Geometry check sheet. Reference: the model listing, model coordinates, mm. Face numbers are marked on the shaded views. A direction names the side the tool comes from. Coordinates: 2 decimals unless noted, no trailing zeros. Loops run counter-clockwise (first coordinate to the right, second up) from the corner with the lowest first, then second, coordinate; pieces in that order, holes last.
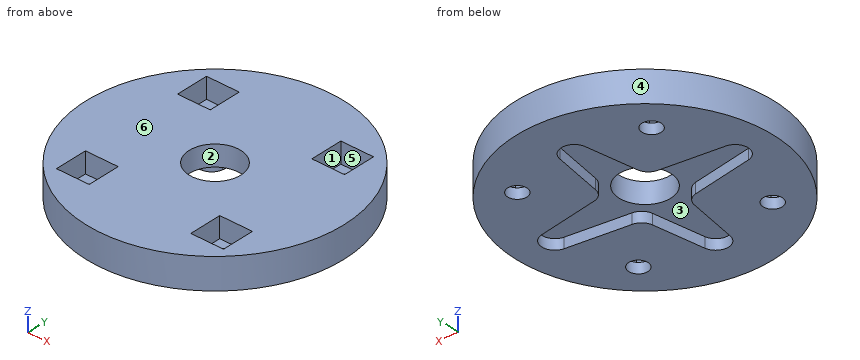
from build123d import *

# Parameters (mm, degrees)
BOSS_EXTRUDE1_OUTLINE_R = 25
BOSS_EXTRUDE1_DEPTH     = 2
SKETCH4_R               = 25
SKETCH4_R_2             = 5
BOSS_EXTRUDE2_DEPTH     = 4
SKETCH5_R               = 1.85
CUT_EXTRUDE1_DEPTH      = 36.860842154
SKETCH6_R               = 3
CUT_EXTRUDE2_DEPTH      = 4
SKETCH7_W               = 6.35
SKETCH7_H               = 6.35
CUT_EXTRUDE3_DEPTH      = 4


# Read off the part's stored shape, not the designer's step: Boss-Extrude1
with BuildPart() as part:
    # Boss-Extrude1 outline → Boss-Extrude1 (new body)
    with BuildSketch(Plane.XY):
        Circle(BOSS_EXTRUDE1_OUTLINE_R)
        with BuildLine():
            ThreePointArc((4.047481829, 6.234173406), (4.763543773, 4.853224592), (6.157606479, 4.163040916))
            Line((6.157606479, 4.163040916), (17.857142857, 2.474358297))
            ThreePointArc((17.857142857, 2.474358297), (20, 0), (17.857142857, -2.474358297))
            Line((17.857142857, -2.474358297), (6.157606479, -4.163040916))
            ThreePointArc((6.157606479, -4.163040916), (4.763543773, -4.853224592), (4.047481829, -6.234173406))
            Line((4.047481829, -6.234173406), (2.467267507, -15.903225806))
            ThreePointArc((2.467267507, -15.903225806), (0, -18), (-2.467267507, -15.903225806))
            Line((-2.467267507, -15.903225806), (-4.047481829, -6.234173406))
            ThreePointArc((-4.047481829, -6.234173406), (-4.763543773, -4.853224592), (-6.157606479, -4.163040916))
            Line((-6.157606479, -4.163040916), (-17.857142857, -2.474358297))
            ThreePointArc((-17.857142857, -2.474358297), (-20, 0), (-17.857142857, 2.474358297))
            Line((-17.857142857, 2.474358297), (-6.157606479, 4.163040916))
            ThreePointArc((-6.157606479, 4.163040916), (-4.763543773, 4.853224592), (-4.047481829, 6.234173406))
            Line((-4.047481829, 6.234173406), (-2.467267507, 15.903225806))
            ThreePointArc((-2.467267507, 15.903225806), (0, 18), (2.467267507, 15.903225806))
            Line((2.467267507, 15.903225806), (4.047481829, 6.234173406))
        make_face(mode=Mode.SUBTRACT)
    extrude(amount=BOSS_EXTRUDE1_DEPTH)

    # Sketch4 → Boss-Extrude2 (add)
    with BuildSketch(Plane.XY.offset(2)):
        Circle(SKETCH4_R)
        Circle(SKETCH4_R_2, mode=Mode.SUBTRACT)
    extrude(amount=BOSS_EXTRUDE2_DEPTH)

    # Sketch5 → Cut-Extrude1 (cut, through all)
    with BuildSketch(Plane.XY.offset(6)):
        with Locations((13.029498672, 13.274798425)):
            Circle(SKETCH5_R)
        with Locations((-13.029498672, 13.274798425)):
            Circle(SKETCH5_R)
        with Locations((-13.029498672, -13.274798425)):
            Circle(SKETCH5_R)
        with Locations((13.029498672, -13.274798425)):
            Circle(SKETCH5_R)
    extrude(amount=-CUT_EXTRUDE1_DEPTH, mode=Mode.SUBTRACT)

    # Sketch6 → Cut-Extrude2 (cut)
    with BuildSketch(Plane.XY.offset(6)):
        with Locations((-13.029498672, -13.274798425)):
            Circle(SKETCH6_R)
        with Locations((13.029498672, -13.274798425)):
            Circle(SKETCH6_R)
        with Locations((13.029498672, 13.274798425)):
            Circle(SKETCH6_R)
        with Locations((-13.029498672, 13.274798425)):
            Circle(SKETCH6_R)
    extrude(amount=-CUT_EXTRUDE2_DEPTH, mode=Mode.SUBTRACT)

    # Sketch7 → Cut-Extrude3 (cut)
    with BuildSketch(Plane.XY.offset(6)):
        with Locations((13.029498672, 13.274798425)):
            Rectangle(SKETCH7_W, SKETCH7_H)
        with Locations((13.029498672, -13.274798425)):
            Rectangle(SKETCH7_W, SKETCH7_H)
        with Locations((-13.029498672, -13.274798425)):
            Rectangle(SKETCH7_W, SKETCH7_H)
        with Locations((-13.029498672, 13.274798425)):
            Rectangle(SKETCH7_W, SKETCH7_H)
    extrude(amount=-CUT_EXTRUDE3_DEPTH, mode=Mode.SUBTRACT)


solid = part.part
1) Mould release check, pull along Y, two halves, no side actions. Record for the marked faces 4, 5 and 6: +Y half, -Y half, draft (parallel to the pull), parting line (faces both ways), or undercut.
Data:
face 4: parting line
face 5: undercut
face 6: draft
2) Section check D-D on y = -8.5. Record the cut outline in (x, z), and give its area (3 significant figures).
Data:
outline: (-23.51, 0) - (-3.68, 0) - (-3.68, 2) - (3.68, 2) - (3.68, 0) - (23.51, 0) - (23.51, 6) - (-23.51, 6) - close
area: 267 mm2
3) Section check C-C on z = 4.3. Record the cut outline in (x, y), and give its area (3 significant figures).
Data:
outline: circle Ø50 at (0, 0); hole (-16.2, -16.45) - (-9.85, -16.45) - (-9.85, -10.1) - (-16.2, -10.1) - close; hole (-16.2, 10.1) - (-9.85, 10.1) - (-9.85, 16.45) - (-16.2, 16.45) - close; hole circle Ø10 at (0, 0); hole (9.85, -16.45) - (16.2, -16.45) - (16.2, -10.1) - (9.85, -10.1) - close; hole (9.85, 10.1) - (16.2, 10.1) - (16.2, 16.45) - (9.85, 16.45) - close
area: 1,720 mm2
4) Depth check by flat-ended pin: pin 1 (2 mm diameter, centred on x = -17, y = 17, fed in from -Z); pin 2 (3 mm diameter, centred on y = -12, z = 3.5, fed in from +X); pin 3 (3 mm diameter, centred on x = -13.03, y = -13.27, fed in from +Z); pin 4 (5 mm diameter, centred on x = -13, y = 13, fed in from +Z). Enter the tip coordinate at first touch or a pass-through.
Data:
pin 1: stops at z = 0
pin 2: stops at x = 22.69
pin 3: passes through
pin 4: stops at z = 2
5) Section check A-A on y = 0. Record the cut outline in (x, z).
Data:
outline: (-25, 0) - (-20, 0) - (-20, 2) - (-5, 2) - (-5, 6) - (-25, 6) - close; (5, 2) - (20, 2) - (20, 0) - (25, 0) - (25, 6) - (5, 6) - close
6) Access from +Z, -Z, +X, -X, +Y, -Y to the whole of each face (thin tool, end or side, straight path). Record for the marked faces 1, 2 and 3.
Data:
face 1: +Z
face 2: +Z, -Z
face 3: -Z
7) Section check B-B on x = 0. Record the cut outline in (y, z).
Data:
outline: (-25, 0) - (-18, 0) - (-18, 2) - (-5, 2) - (-5, 6) - (-25, 6) - close; (5, 2) - (18, 2) - (18, 0) - (25, 0) - (25, 6) - (5, 6) - close
8) Material ranges on probe 1 along Y at (x, z) = (-13, 3.35); probe 2 along Y at (x, z) = (12, 1.1); probe 3 along Z at (x, y) = (-16, 2), recorded low to high.
Data:
probe 1: y = -21.35 to -16.45, -10.1 to 10.1, 16.45 to 21.35
probe 2: y = -21.93 to -14.81, -11.74 to -3.32, 3.32 to 11.74, 14.81 to 21.93
probe 3: z = 2 to 6
